The drawing under review shows one solid part. Ordinate dimensions are in mm from its lowest x, y, z. A direction names the side the tool comes from. Give positions to 0.01 mm unless a question says otherwise; leave off trailing zeros. Write each loop counter-clockwise with the first axis right and the second up, starting at its lowest first coordinate (ties: lowest second). Pieces come first, ordered by that corner, then holes. Notation, with made-up numbers: (1, -16.75) -> (52, -16.75) arc R20 ccw to (52, 10.25) -> close; hole circle Ø1 at (27.5, -16). An arc over 180 degrees is marked (long way). Write item = value, one per line.
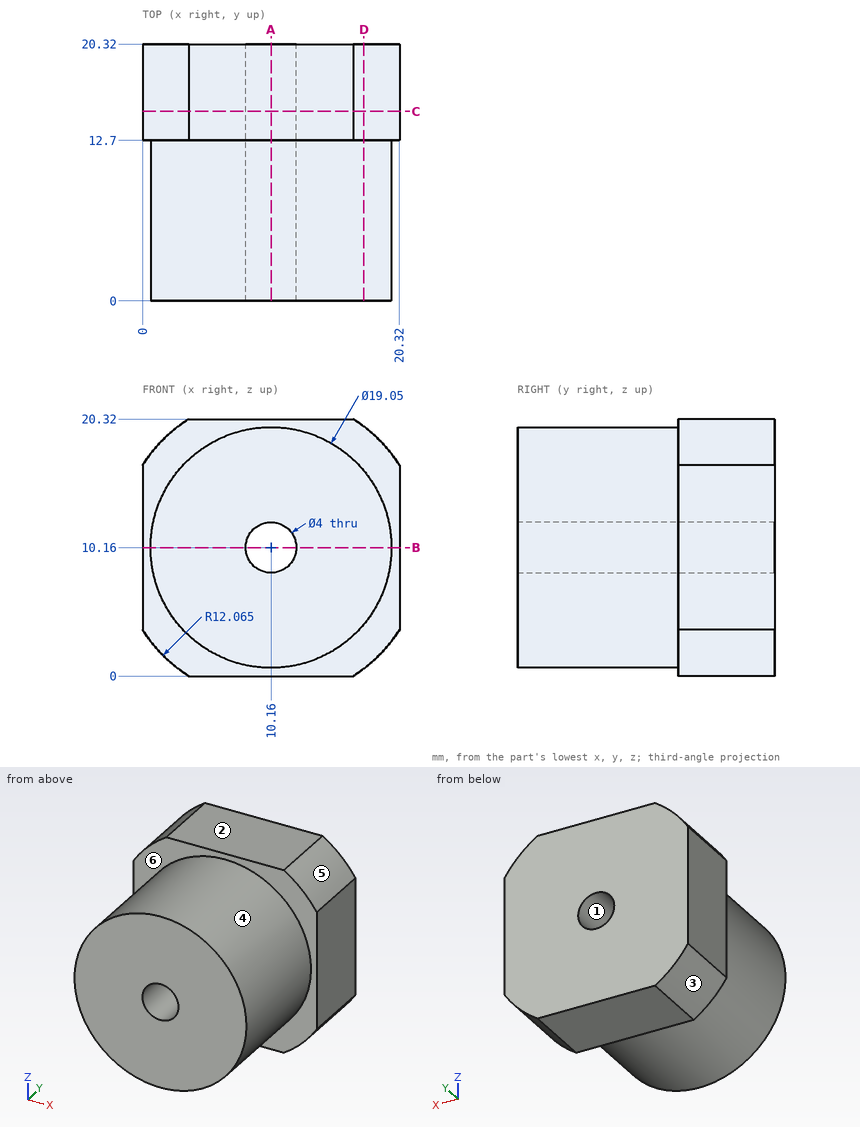
(1) Take a section at A-A (x = 10.16). Write out the cut boundary in (y, z) (3 decimals).
Answers below:
outline = (0, 0.635) -> (12.7, 0.635) -> (12.7, 0) -> (20.32, 0) -> (20.32, 8.16) -> (0, 8.16) -> close; (0, 12.16) -> (20.32, 12.16) -> (20.32, 20.32) -> (12.7, 20.32) -> (12.7, 19.685) -> (0, 19.685) -> close
(2) To check wall thickness, follow probe 1 along X at (y, z) = (10.75, 10.16) (3 decimals); probe 2 along X at (y, z) = (13, 10.16); probe 3 along X at (y, z) = (1.5, 16.25). State the ranges of each line that lie inside material, in increasing order.
Answers below:
probe_1 = 0.635 to 8.16, 12.16 to 19.685
probe_2 = 0 to 8.16, 12.16 to 20.32
probe_3 = 2.84 to 17.48
(3) The part is to be moulded in two halves that separate along Z. For the marked faces 1, 2, 3 and 4, say which applies: released by +Z, released by -Z, zero draft, split by the parting line, or undercut.
Answers below:
face_1 = undercut
face_2 = released by +Z
face_3 = released by -Z
face_4 = split by the parting line
(4) Take a section at C-C (y = 15). Write out the cut boundary in (x, z) (3 decimals).
Answers below:
outline = (0, 3.653) arc R12.065 ccw to (3.653, 0) -> (16.667, 0) arc R12.065 ccw to (20.32, 3.653) -> (20.32, 16.667) arc R12.065 ccw to (16.667, 20.32) -> (3.653, 20.32) arc R12.065 ccw to (0, 16.667) -> close; hole circle Ø4 at (10.16, 10.16)
(5) Take a section at B-B (z = 10.16). Write out the cut boundary in (x, y) (3 decimals).
Answers below:
outline = (0, 12.7) -> (0.635, 12.7) -> (0.635, 0) -> (8.16, 0) -> (8.16, 20.32) -> (0, 20.32) -> close; (12.16, 0) -> (19.685, 0) -> (19.685, 12.7) -> (20.32, 12.7) -> (20.32, 20.32) -> (12.16, 20.32) -> close
(6) Tool access review of the marked faces 5 and 6: name each direction out of +Z, -Z, +X, -X, +Y, -Y from which nothing blocks a thin tool from reaching the whole face with its end or side.
Answers below:
face_5 = +Z, +X, +Y, -Y
face_6 = -Y
(7) Take a section at D-D (x = 17.5). Write out the cut boundary in (y, z), plus the area to 3 significant figures.
Answers below:
outline = (0, 4.09) -> (12.7, 4.09) -> (12.7, 0.58) -> (20.32, 0.58) -> (20.32, 19.74) -> (12.7, 19.74) -> (12.7, 16.23) -> (0, 16.23) -> close
area = 300 mm^2
(8) For pin 1 (6 mm diameter, centred on x = 9, y = 5, fed in from +Z) (3 decimals); pin 2 (2 mm diameter, centred on y = 10.5, z = 18, fed in from +X); pin 3 (1 mm diameter, centred on x = 3, y = 8, fed in from -Z), all flat-tipped, find the tip position at first contact; note any pin that passes through.
Answers below:
pin_1 = 19.685
pin_2 = 16.79
pin_3 = 3.35
